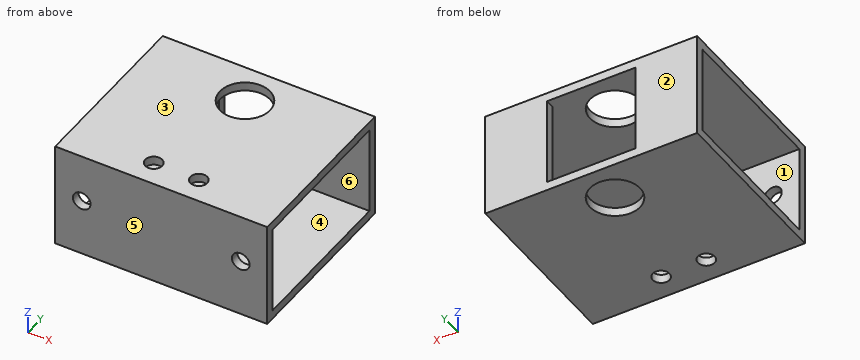
```python
from build123d import *

# Parameters (mm, degrees)
SKETCH1_W           = 38.1
SKETCH1_H           = 63.5
SKETCH1_W_2         = 31.75
SKETCH1_H_2         = 57.15
BOSS_EXTRUDE1_DEPTH = 76.2
SKETCH2_R           = 9
SKETCH2_R_2         = 3.025
CUT_EXTRUDE1_DEPTH  = 38.1
SKETCH3_W           = 31.75
SKETCH3_H           = 31.75
CUT_EXTRUDE2_DEPTH  = 76.2
SKETCH4_R           = 3.175
CUT_EXTRUDE3_DEPTH  = 32.75


with BuildPart() as part:
    # Sketch1 → Boss-Extrude1 (new body)
    with BuildSketch(Plane(origin=(0, 0, 0), x_dir=(0, 0, -1), z_dir=(1, 0, 0))):
        Rectangle(SKETCH1_W, SKETCH1_H)
        Rectangle(SKETCH1_W_2, SKETCH1_H_2, mode=Mode.SUBTRACT)
    extrude(amount=BOSS_EXTRUDE1_DEPTH)

    # Sketch2 → Cut-Extrude1 (cut, symmetric)
    with BuildSketch(Plane.XY):
        with Locations((38.1, 17.7)):
            Circle(SKETCH2_R)
        with Locations((46.205, -22.86)):
            Circle(SKETCH2_R_2)
        with Locations((29.995, -22.86)):
            Circle(SKETCH2_R_2)
    extrude(amount=CUT_EXTRUDE1_DEPTH, both=True, mode=Mode.SUBTRACT)

    # Sketch3 → Cut-Extrude2 (cut)
    with BuildSketch(Plane(origin=(0, 0, 0), x_dir=(1, 0, 0), z_dir=(0, 1, 0))):
        with Locations((38.1, 0)):
            Rectangle(SKETCH3_W, SKETCH3_H)
    extrude(amount=CUT_EXTRUDE2_DEPTH, mode=Mode.SUBTRACT)

    # Sketch4 → Cut-Extrude3 (cut, through all)
    with BuildSketch(Plane(origin=(0, 0, 0), x_dir=(1, 0, 0), z_dir=(0, 1, 0))):
        with Locations((9.525, -1.5875)):
            Circle(SKETCH4_R)
        with Locations((66.675, -1.5875)):
            Circle(SKETCH4_R)
    extrude(amount=-CUT_EXTRUDE3_DEPTH, mode=Mode.SUBTRACT)


solid = part.part
```
Model file for the job. Use its own axes, mm. Face numbers are marked on the shaded views. A direction names the side the tool comes from. Coordinates: 2 decimals unless noted, no trailing zeros. Order: outer loops, then holes, each group sorted by start corner. A loop starts at its lowest first (then second) coordinate and runs counter-clockwise, first axis right, second up. Notation, with made-up numbers: (-16, 51.25) -> (40, 51.25) arc R19 cw to (40, 62.25) -> close; hole circle Ø2 at (-35.75, -2). An arc over 180 degrees is marked (long way). Answer as a JSON object with one key per item and string values. Group by question number.
1) Which spindle directions (+Z, -Z, +X, -X, +Y, -Y) get a long thin tool onto all of the face, cutting with end or side? Do the marked faces 5 and 6. Say none if no direction does.
2) Cut at C-C, the plane z = 12. Write the cut outline in (x, y) (3 decimals).
3) Drill centre lines: L1, parallel to Y at x = 4, z = -6 (3 decimals); L2, parallel to X at y = 17.7, z = 17.3; L3, parallel to Z at x = 31.5, y = 3 (3 decimals). Where is each one in solid material? Low to high.
4) Cut at A-A, the plane y = -22.86. Write the cut outline in (x, z) (3 decimals), then the cut area to 3 significant figures.
5) Cut at D-D, the plane y = 4.5. Write the cut outline in (x, z) (3 decimals), then the cut area to 3 significant figures.
6) Cut at B-B, the plane x = 38.1. Write the cut outline in (y, z) (3 decimals).
7) Pull direction Y, two halves, no side cores. Call the marked faces 1, 2, 3 and 4: +Y half, -Y half, draft (parallel to the pull), parting line (faces both ways), or undercut.
8) Flat gauge pins, fed straight in: pin 1 (5 mm diameter, centred on x = 29.995, y = -22.86, fed in from -Z); pin 2 (1.5 mm diameter, centred on x = 37, z = 7, fed in from +Y) (3 decimals). Where does each tip first touch, or does it go through?
Check values:
{
 "1": {"face 5": "+Z, -Z, +X, -X, -Y", "face 6": "+X, -X"},
 "2": {"outline": "(0, -31.75) -> (76.2, -31.75) -> (76.2, -28.575) -> (0, -28.575) -> close; (0, 28.575) -> (22.225, 28.575) -> (22.225, 31.75) -> (0, 31.75) -> close; (53.975, 28.575) -> (76.2, 28.575) -> (76.2, 31.75) -> (53.975, 31.75) -> close"},
 "3": {"L1": "y = -31.75 to -28.575, 28.575 to 31.75", "L2": "x = 0 to 29.1, 47.1 to 76.2", "L3": "z = -19.05 to -15.875, 15.875 to 19.05"},
 "4": {"outline": "(0, -19.05) -> (26.97, -19.05) -> (26.97, -15.875) -> (0, -15.875) -> close; (0, 15.875) -> (26.97, 15.875) -> (26.97, 19.05) -> (0, 19.05) -> close; (33.02, -19.05) -> (43.18, -19.05) -> (43.18, -15.875) -> (33.02, -15.875) -> close; (33.02, 15.875) -> (43.18, 15.875) -> (43.18, 19.05) -> (33.02, 19.05) -> close; (49.23, -19.05) -> (76.2, -19.05) -> (76.2, -15.875) -> (49.23, -15.875) -> close; (49.23, 15.875) -> (76.2, 15.875) -> (76.2, 19.05) -> (49.23, 19.05) -> close", "area": "407 mm²"},
 "5": {"outline": "(0, -19.05) -> (76.2, -19.05) -> (76.2, -15.875) -> (0, -15.875) -> close; (0, 15.875) -> (76.2, 15.875) -> (76.2, 19.05) -> (0, 19.05) -> close", "area": "484 mm²"},
 "6": {"outline": "(-31.75, -19.05) -> (8.7, -19.05) -> (8.7, -15.875) -> (-28.575, -15.875) -> (-28.575, 15.875) -> (8.7, 15.875) -> (8.7, 19.05) -> (-31.75, 19.05) -> close; (26.7, -19.05) -> (31.75, -19.05) -> (31.75, -15.875) -> (26.7, -15.875) -> close; (26.7, 15.875) -> (31.75, 15.875) -> (31.75, 19.05) -> (26.7, 19.05) -> close"},
 "7": {"face 1": "undercut", "face 2": "+Y half", "face 3": "draft", "face 4": "undercut"},
 "8": {"pin 1": "passes through", "pin 2": "stops at y = -28.575"}
}
